Source: CAD feature listing. Evaluate the final solid. Frame: model axes, mm. A direction names the side the tool comes from. Coordinates: 2 decimals unless noted, no trailing zeros. Loops run counter-clockwise (first coordinate to the right, second up) from the corner with the lowest first, then second, coordinate; pieces in that order, holes last. Notation, with made-up numbers: (58, -16.75) - (67, -16.75) arc R15 ccw to (67, 1.25) - close; hole circle Ø8 at (87, 18). An arc over 180 degrees is marked (long way). Write item = value, one per line. Start each with the question number.
from build123d import *

# Parameters (mm, degrees)
SKETCH1_W               = 50
SKETCH1_H               = 50
BOSS_EXTRUDE1_DEPTH     = 200
SKETCH4_W               = 30
SKETCH4_H               = 50
CUT_EXTRUDE1_DEPTH      = 80
CUT_EXTRUDE2_DEPTH      = 213.132034356
CUT_EXTRUDE2_DEPTH_BACK = 213.132034356


with BuildPart() as part:
    # Sketch1 → Boss-Extrude1 (new body)
    with BuildSketch(Plane(origin=(0, 0, 0), x_dir=(1, 0, 0), z_dir=(0, 1, 0))):
        with Locations((-25, 25)):
            Rectangle(SKETCH1_W, SKETCH1_H)
    extrude(amount=BOSS_EXTRUDE1_DEPTH)

    # Sketch4 → Cut-Extrude1 (cut)
    with BuildSketch(Plane(origin=(0, 200, 0), x_dir=(1, 0, 0), z_dir=(0, 1, 0))):
        with Locations((-25, 25)):
            Rectangle(SKETCH4_W, SKETCH4_H)
    extrude(amount=-CUT_EXTRUDE1_DEPTH, mode=Mode.SUBTRACT)

    # Sketch5 → Cut-Extrude2 (cut, two sides: drawn at the far end of the back side and taken through both)
    with BuildSketch(Plane(origin=(0, 0, 0), x_dir=(0, 0, -1), z_dir=(1, 0, 0)).offset(-CUT_EXTRUDE2_DEPTH_BACK)):
        with BuildLine():
            Line((-217.391133594, -142.729464946), (0, 185))
            ThreePointArc((0, 185), (25, 198.416876048), (50, 185))
            Line((50, 185), (267.391133594, -142.729464946))
            Line((267.391133594, -142.729464946), (267.391133594, 643.821250924))
            Line((267.391133594, 643.821250924), (-217.391133594, 643.821250924))
            Line((-217.391133594, 643.821250924), (-217.391133594, -142.729464946))
        make_face()
    extrude(amount=CUT_EXTRUDE2_DEPTH + CUT_EXTRUDE2_DEPTH_BACK, mode=Mode.SUBTRACT)


solid = part.part
Item 1: Reachability of faces 4 (the flat face through (-40, 160, -25)), 5 (the flat face through (-25, 0, -25)) from +Z, -Z, +X, -X, +Y, -Y: full face, straight path, thin tool, end or side. Return the list, or none.
Item 2: Cut plane B-B (z = -20.5). Return the cut outline in (x, y).
Item 3: Material intervals for L1, parallel to Y at x = -23.5, z = -2; L2, parallel to X at y = 151.5, z = -14.5; L3, parallel to Y at x = -47, z = -32.5, sorted ascending. Write a range as [from, to].
Item 4: Draft query along X for faces 1 (the flat face through (-25, 120, -25)), 2 (the flat face through (-50, 98, -25)), 3 (the flat face through (-25, 71, 0)). Return one class per face: released by +X, released by -X, zero draft, split by the parting line, or undercut.
Item 5: Cut plane A-A (y = 161). Return the cut outline in (x, z).
Item 6: Cut plane D-D (z = -33). Return the cut outline in (x, y).
Item 7: First-contact query: pin 1 (4 mm diameter, centred on y = 149.5, z = -17, fed in from +X); pin 2 (9 mm diameter, centred on x = -25.5, z = -31, fed in from +Y). Flat tips, straight axial feed; report the tip coordinate or a pass-through.
Item 8: Cut plane C-C (x = -30.5). Return the cut outline in (y, z), then the cut area to 3 significant figures.
Responses:
q1.face_4 = +Z, -Z, +Y
q1.face_5 = +Z, -Z, +X, -X, -Y
q2.outline = (-50, 0) - (0, 0) - (0, 198.08) - (-10, 198.08) - (-10, 120) - (-40, 120) - (-40, 198.08) - (-50, 198.08) - close
q3.L1 = [0, 120]
q3.L2 = [-50, -40], [-10, 0]
q3.L3 = [0, 197.46]
q4.face_1 = undercut
q4.face_2 = released by -X
q4.face_3 = zero draft
q5.outline = (-50, -50) - (-40, -50) - (-40, 0) - (-50, 0) - close; (-10, -50) - (0, -50) - (0, 0) - (-10, 0) - close
q6.outline = (-50, 0) - (0, 0) - (0, 197.33) - (-10, 197.33) - (-10, 120) - (-40, 120) - (-40, 197.33) - (-50, 197.33) - close
q7.pin_1 = 0
q7.pin_2 = 120
q8.outline = (0, -50) - (120, -50) - (120, 0) - (0, 0) - close
q8.area = 6,000 mm2
